Answer from the drawing. Dimensions are ordinates in mm from the lowest x, y and z of the part. A direction names the side the tool comes from. Round coordinates to 2 decimals unless told otherwise and drop trailing zeros. Loops run counter-clockwise (first coordinate to the right, second up) from the corner with the lowest first, then second, coordinate; pieces in that order, holes last. Notation, with made-up numbers: (41, 12) - (95, 12) arc R20 ccw to (95, 32) - close; hole circle Ø4 at (26.25, 11.25). An arc over 180 degrees is marked (long way). Return JSON: item names as keys, results as strings.
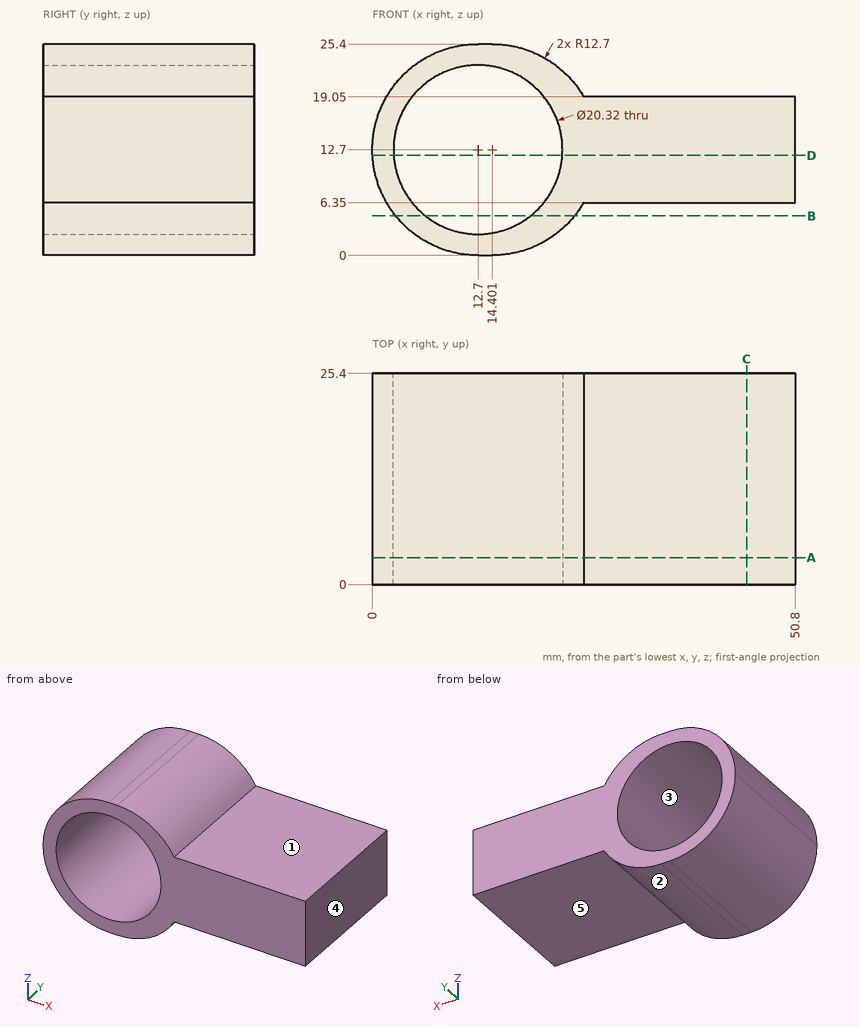
1) Flat-ended cylindrical pins translate along their axes: pin 1 (5 mm diameter, centred on x = 41.5, y = 16, fed in from -Z); pin 2 (8 mm diameter, centred on y = 4, z = 21, fed in from +X); pin 3 (12 mm diameter, centred on x = 12.7, z = 12.7, fed in from -Y); pin 4 (2 mm diameter, centred on x = 39.5, y = 14, fed in from +Z). Find the tip coordinate at first contact, or state that the pin passes through.
Verdict:
{"pin 1": "stops at z = 6.35", "pin 2": "stops at x = 50.8", "pin 3": "passes through", "pin 4": "stops at z = 19.05"}
2) Find the intervals of material crossed by L1, parallel to Z at x = 35.5, y = 7.25; L2, parallel to Z at x = 13, y = 20 (1 decimal); L3, parallel to X at y = 12, z = 10 (1 decimal), in increasing order.
Verdict:
{"L1": "z = 6.35 to 19.05", "L2": "z = 0 to 2.5, 22.9 to 25.4", "L3": "x = 0.3 to 2.9, 22.5 to 50.8"}
3) Section A-A (y = 3.25) is taken. Give the vertices of the cut face in (x, z).
Verdict:
{"outline": "(12.7, 0) - (14.4, 0) arc R12.7 ccw to (25.4, 6.35) - (50.8, 6.35) - (50.8, 19.05) - (25.4, 19.05) arc R12.7 ccw to (14.4, 25.4) - (12.7, 25.4) arc R12.7 ccw to start; hole circle Ø20.32 at (12.7, 12.7)"}
4) Section D-D (z = 12) is taken. Give the vertices of the cut face in (x, y) (1 decimal), and give its area (3 significant figures).
Verdict:
{"outline": "(0, 0) - (2.6, 0) - (2.6, 25.4) - (0, 25.4) - close; (22.8, 0) - (50.8, 0) - (50.8, 25.4) - (22.8, 25.4) - close", "area": "775 mm2"}
5) Section C-C (x = 45) is taken. Give the vertices of the cut face in (y, z), and give its area (3 significant figures).
Verdict:
{"outline": "(0, 6.35) - (25.4, 6.35) - (25.4, 19.05) - (0, 19.05) - close", "area": "323 mm2"}
6) Determine the mould class of the marked faces 3, 4 and 5 for opening direction X: pulls with the +X half, pulls with the -X half, needs draft (parallel to the pull), parting line crosses it, or undercut.
Verdict:
{"face 3": "undercut", "face 4": "pulls with the +X half", "face 5": "needs draft"}
7) Section B-B (z = 4.75) is taken. Give the vertices of the cut face in (x, y) (1 decimal).
Verdict:
{"outline": "(2.8, 0) - (6.4, 0) - (6.4, 25.4) - (2.8, 25.4) - close; (19, 0) - (24.3, 0) - (24.3, 25.4) - (19, 25.4) - close"}
8) A tool of negligible diameter and unlimited length cuts with its end or side. For the marked faces 1 and 2, from which of +Z, -Z, +X, -X, +Y, -Y can it reach the whole face along a straight path? Write none if from no direction.
Verdict:
{"face 1": "+Z, +X, +Y, -Y", "face 2": "-Z, +X, +Y, -Y"}
